Part model, mm, in its own coordinate system. Face numbers are marked on the shaded views. A direction names the side the tool comes from. Give positions to 0.01 mm unless a question says otherwise; leave off trailing zeros. Write each loop counter-clockwise with the first axis right and the second up, starting at its lowest first coordinate (ties: lowest second). Pieces come first, ordered by that corner, then holes.
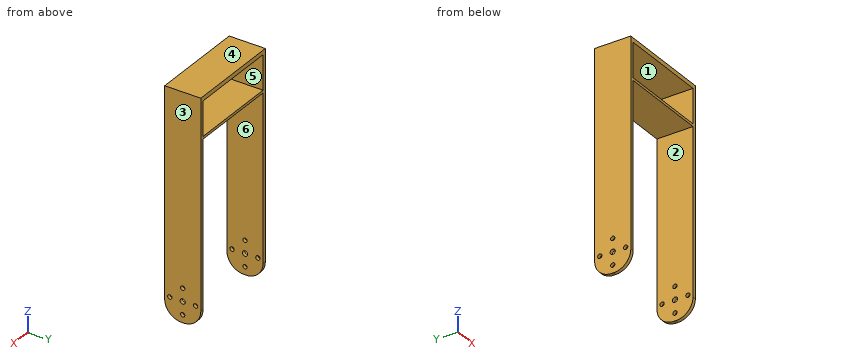
from build123d import *

# Parameters (mm, degrees)
SKETCH3_W           = 56
SKETCH3_H           = 21
BOSS_EXTRUDE1_DEPTH = 130
SKETCH4_W           = 52
SKETCH4_H           = 106
SKETCH4_H_2         = 20
CUT_EXTRUDE3_DEPTH  = 22
SKETCH6_R           = 1.5
SKETCH6_R_2         = 1.25
CUT_EXTRUDE4_DEPTH  = 57
FILLET1_R           = 10


with BuildPart() as part:
    # Sketch3 → Boss-Extrude1 (new body)
    with BuildSketch(Plane.XY):
        Rectangle(SKETCH3_W, SKETCH3_H)
    extrude(amount=BOSS_EXTRUDE1_DEPTH)

    # Sketch4 → Cut-Extrude3 (cut, through all)
    with BuildSketch(Plane.XZ.offset(10.5)):
        with Locations((0, 53)):
            Rectangle(SKETCH4_W, SKETCH4_H)
        with Locations((0, 117.5)):
            Rectangle(SKETCH4_W, SKETCH4_H_2)
    extrude(amount=-CUT_EXTRUDE3_DEPTH, mode=Mode.SUBTRACT)

    # Sketch6 → Cut-Extrude4 (cut, through all)
    with BuildSketch(Plane(origin=(28, 0, 0), x_dir=(0, 0, -1), z_dir=(1, 0, 0))):
        with Locations((-12, 0)):
            Circle(SKETCH6_R)
        with Locations((-4.5, 0)):
            Circle(SKETCH6_R_2)
        with Locations((-19.5, 0)):
            Circle(SKETCH6_R_2)
        with Locations((-12, 7.5)):
            Circle(SKETCH6_R_2)
        with Locations((-12, -7.5)):
            Circle(SKETCH6_R_2)
    extrude(amount=-CUT_EXTRUDE4_DEPTH, mode=Mode.SUBTRACT)

    # Fillet1
    fillet1_edges = [part.edges().sort_by_distance(p)[0] for p in [
        (27, -10.5, 0),
        (-27, 10.5, 0),
        (-27, -10.5, 0),
        (27, 10.5, 0),
    ]]
    fillet(fillet1_edges, radius=FILLET1_R)


solid = part.part
1) Saw through at C-C (x = 15). Write the cut outline in (y, z), and give its area (3 significant figures).
Check result:
outline: (-10.5, 106) - (10.5, 106) - (10.5, 107.5) - (-10.5, 107.5) - close; (-10.5, 127.5) - (10.5, 127.5) - (10.5, 130) - (-10.5, 130) - close
area: 84.0 mm2
2) Saw through at A-A (z = 19.5). Write the cut outline in (x, y).
Check result:
outline: (-28, -10.5) - (-26, -10.5) - (-26, -1.25) - (-28, -1.25) - close; (-28, 1.25) - (-26, 1.25) - (-26, 10.5) - (-28, 10.5) - close; (26, -10.5) - (28, -10.5) - (28, -1.25) - (26, -1.25) - close; (26, 1.25) - (28, 1.25) - (28, 10.5) - (26, 10.5) - close
3) 3-axis set-ups, long thin cutter, end or side, ignore diameter. For the marked faces 1, 2 and 3: which of +Z, -Z, +X, -X, +Y, -Y reach the whole face in a straight line?
Check result:
face 1: +Y, -Y
face 2: -Z, +Y, -Y
face 3: +Z, -Z, +X, +Y, -Y
4) Flat gauge pins, fed straight in: P1, Ø1.5, axis at y = -7.5, z = 12, coming from the +X side; P2, Ø2, axis at x = -4, y = 6, coming from the -Z side. Where does each tip first touch, or does it go through?
Check result:
P1: passes through
P2: stops at z = 106
5) Saw through at B-B (z = 52.5). Write the cut outline in (x, y).
Check result:
outline: (-28, -10.5) - (-26, -10.5) - (-26, 10.5) - (-28, 10.5) - close; (26, -10.5) - (28, -10.5) - (28, 10.5) - (26, 10.5) - close
6) Mould opens along Z. For the marked faces 4, 5 and 6 say: +Z half, -Z half, draft (parallel to the pull), parting line (faces both ways), or undercut.
Check result:
face 4: +Z half
face 5: undercut
face 6: draft
7) Drill centre lines: L1, parallel to Y at x = -26.7, z = 12; L2, parallel to X at y = -9, z = 69.5; L3, parallel to Z at x = 15, y = 0.25. Where is each one in solid material? Low to high.
Check result:
L1: y = -10.5 to -8.75, -6.25 to -1.5, 1.5 to 6.25, 8.75 to 10.5
L2: x = -28 to -26, 26 to 28
L3: z = 106 to 107.5, 127.5 to 130
8) Saw through at D-D (y = 7.5). Write the cut outline in (x, z).
Check result:
outline: (-28, 2.86) - (-26, 2.86) - (-26, 10.75) - (-28, 10.75) - close; (-28, 13.25) - (-26, 13.25) - (-26, 106) - (26, 106) - (26, 13.25) - (28, 13.25) - (28, 130) - (-28, 130) - close; (26, 2.86) - (28, 2.86) - (28, 10.75) - (26, 10.75) - close; hole (-26, 107.5) - (26, 107.5) - (26, 127.5) - (-26, 127.5) - close
